The drawing under review shows one solid part. Ordinate dimensions are in mm from its lowest x, y, z. A direction names the side the tool comes from. Coordinates: 2 decimals unless noted, no trailing zeros. Order: outer loops, then holes, each group sorted by start corner. A loop starts at its lowest first (then second) coordinate and runs counter-clockwise, first axis right, second up. Notation, with made-up numbers: (-8.75, 64) -> (46.25, 64) arc R15 cw to (46.25, 74) -> close; hole circle Ø2 at (25.5, -5). An arc over 180 degrees is marked (long way). Write item = value, one per line.
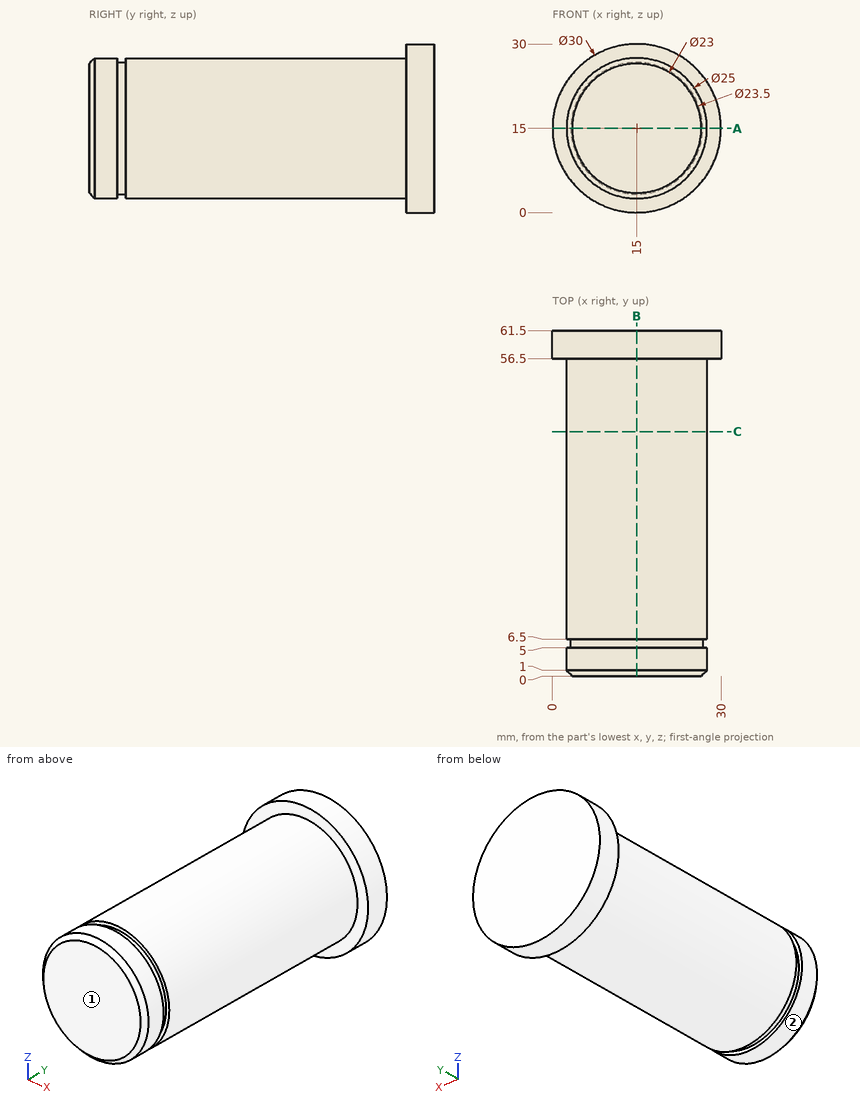
(1) For the marked faces 1 and 2, list the 3-axis set-ups (+Z, -Z, +X, -X, +Y, -Y) from which the entire face can be reached by the end or side of a thin tool; tool diameter is ignored.
Report:
face_1 = +Z, -Z, +X, -X, -Y
face_2 = -Y
(2) We need section C-C (y = 43.5). Write out the cut boundary in (x, z).
Report:
outline = circle Ø25 at (15, 15)
(3) Insertion check: pin 1 (12 mm diameter, centred on x = 25, y = 47, fed in from +Z); pin 2 (2 mm diameter, centred on y = 44, z = 8.5, fed in from -X) (3 decimals); pin 3 (2 mm diameter, centred on y = 48.5, z = 24.5, fed in from -X). Each pin has a flat end and moves straight along its axis. Give the tip position at first contact, or say it passes through.
Report:
pin_1 = 26.84
pin_2 = 3.775
pin_3 = 5.83
(4) We need section B-B (x = 15). Write out the cut boundary in (y, z).
Report:
outline = (0, 3.5) -> (1, 2.5) -> (5, 2.5) -> (5, 3.25) -> (6.5, 3.25) -> (6.5, 2.5) -> (56.5, 2.5) -> (56.5, 0) -> (61.5, 0) -> (61.5, 30) -> (56.5, 30) -> (56.5, 27.5) -> (6.5, 27.5) -> (6.5, 26.75) -> (5, 26.75) -> (5, 27.5) -> (1, 27.5) -> (0, 26.5) -> close
(5) For L1, parallel to Z at x = 15.25, y = 42; L2, parallel to Y at x = 7.5, z = 3.5; L3, parallel to Z at x = 18.75, y = 15, list the stretches that pass through material, from the lowest coordinate up.
Report:
L1 = 2.5 to 27.5
L2 = 56.5 to 61.5
L3 = 3.08 to 26.92
(6) We need section A-A (z = 15). Write out the cut boundary in (x, y), and give its area (3 significant figures).
Report:
outline = (0, 56.5) -> (2.5, 56.5) -> (2.5, 6.5) -> (3.25, 6.5) -> (3.25, 5) -> (2.5, 5) -> (2.5, 1) -> (3.5, 0) -> (26.5, 0) -> (27.5, 1) -> (27.5, 5) -> (26.75, 5) -> (26.75, 6.5) -> (27.5, 6.5) -> (27.5, 56.5) -> (30, 56.5) -> (30, 61.5) -> (0, 61.5) -> close
area = 1,560 mm²
